The model under review builds one solid part; all positions refer to its coordinate system, in mm. A direction names the side the tool comes from. Coordinates: 2 decimals unless noted, no trailing zeros. Loops run counter-clockwise (first coordinate to the right, second up) from the corner with the lowest first, then second, coordinate; pieces in that order, holes last. Notation, with made-up numbers: M 83,36.25 L 134,36.25 A35 cw 134,74.25 Z; hole C 45.5,62.5 d6. An arc over 180 degrees is marked long. Write item = value, one per line. Start each with the question number.
Q1. We need section B-B on x = 0. Count the separate pieces of the cut face and the enclosed holes in it, and give its area (3 significant figures).
Q2. We need section C-C on y = 26. Give the boundary of the cut face in (x, z), and give its area (3 significant figures).
Q3. Mouldability with a two-part tool opening along X and no side actions: class faces 4 (the face through (-1.11, 16.01, 1.27)), 5 (the face through (-5, 15, 2)), 6 (the face through (0, 0, 1)) as released by +X, released by -X, zero draft, split by the parting line, or undercut.
Q4. For faces 1 (the face through (0, 9, 2.5)), 2 (the face through (5, 15, 2)), 3 (the face through (-0.03, 2.25, 1.27)), list the 3-axis set-ups (+Z, -Z, +X, -X, +Y, -Y) from which the entire face can be reached by the end or side of a thin tool; tool diameter is ignored.
Q5. Wall thickness on probe 1 along Y at (x, z) = (0, 1.85); probe 2 along Y at (x, z) = (0, 0.95); probe 3 along Z at (x, y) = (3, 11): over which ranges is each line inside the solid? List them lowest first.
Q6. Clearance check with flat-ended pins moving along their axes: pin 1 Ø4 at (x, y) = (1.5, 7.5) entering from +Z; pin 2 Ø2 at (x, y) = (-3.5, 21.5) entering from -Z. State where each tip first meets the part, or that it passes through.
Q7. We need section D-D on z = 7.5. Give the boundary of the cut face in (x, y), and give its area (3 significant figures).
Q8. We need section A-A on y = 15. Give the boundary of the cut face in (x, z), and give its area (3 significant figures).
from build123d import *

# Parameters (mm, degrees)
F1_DEPTH      = 5
F1_DEPTH_BACK = 5
F2_R          = 3
F3_R          = 3
F4_R          = 1.5
F5_DEPTH      = 2.5


with BuildPart() as f1:
    # F0 (on Right) → F1 (new body, two sides)
    with BuildSketch(Plane.YZ) as f1_sk:
        Polygon((0, 2.5), (0, 0), (21, 0), (24, 4), (22, 5.5), (19.75, 2.5), align=None)
        Polygon((22, 5.5), (24, 4), (30, 6), (29.209430585, 8.3717082451), (22.4685647168, 6.1247529557), align=None)
    extrude(amount=F1_DEPTH)
    extrude(f1_sk.sketch, amount=-F1_DEPTH_BACK)

    # F2
    f2_edges = [f1.edges().sort_by_distance(p)[0] for p in [
        (0, 21, 0),
        (0, 19.75, 2.5),
    ]]
    fillet(f2_edges, radius=F2_R)

    # F3
    f3_edges = [f1.edges().sort_by_distance(p)[0] for p in [
        (0, 22.468565, 6.124753),
        (0, 24, 4),
    ]]
    fillet(f3_edges, radius=F3_R)

    # F4 (on face) → F5 (cut, through all)
    with BuildSketch(Plane.XY.offset(2.5)):
        with Locations((0, 15)):
            Circle(F4_R)
        with BuildLine():
            ThreePointArc((1.4947825929, 3.875), (1.4986950806, 3.937445581), (1.5, 4))
            ThreePointArc((1.5, 4), (1.4986950806, 4.062554419), (1.4947825929, 4.125))
            ThreePointArc((1.4947825929, 4.125), (1.4882142436, 4.0623344324), (1.4790199458, 4))
            ThreePointArc((1.4790199458, 4), (1.4882142436, 3.9376655676), (1.4947825929, 3.875))
        make_face()
        with BuildLine():
            ThreePointArc((-1.4790199458, 4), (-1.4882142436, 4.0623344324), (-1.4947825929, 4.125))
            ThreePointArc((-1.4947825929, 4.125), (-1.4986950806, 4.062554419), (-1.5, 4))
            ThreePointArc((-1.5, 4), (-1.4986950806, 3.937445581), (-1.4947825929, 3.875))
            ThreePointArc((-1.4947825929, 3.875), (-1.4882142436, 3.9376655676), (-1.4790199458, 4))
        make_face()
        with BuildLine():
            ThreePointArc((-1.4790199458, 4), (0, 2.75), (1.4790199458, 4))
            ThreePointArc((1.4790199458, 4), (0, 5.25), (-1.4790199458, 4))
        make_face()
        with BuildLine():
            ThreePointArc((1.4790199458, 4), (1.4882142436, 4.0623344324), (1.4947825929, 4.125))
            ThreePointArc((1.4947825929, 4.125), (0, 5.5), (-1.4947825929, 4.125))
            ThreePointArc((-1.4947825929, 4.125), (-1.4882142436, 4.0623344324), (-1.4790199458, 4))
            ThreePointArc((-1.4790199458, 4), (0, 5.25), (1.4790199458, 4))
        make_face()
        with BuildLine():
            ThreePointArc((-1.4947825929, 4.125), (0, 5.5), (1.4947825929, 4.125))
            ThreePointArc((1.4947825929, 4.125), (1.4986950806, 4.187445581), (1.5, 4.25))
            ThreePointArc((1.5, 4.25), (0, 5.75), (-1.5, 4.25))
            ThreePointArc((-1.5, 4.25), (-1.4986950806, 4.187445581), (-1.4947825929, 4.125))
        make_face()
        with BuildLine():
            ThreePointArc((-1.4947825929, 3.875), (0, 2.5), (1.4947825929, 3.875))
            ThreePointArc((1.4947825929, 3.875), (1.4882142436, 3.9376655676), (1.4790199458, 4))
            ThreePointArc((1.4790199458, 4), (0, 2.75), (-1.4790199458, 4))
            ThreePointArc((-1.4790199458, 4), (-1.4882142436, 3.9376655676), (-1.4947825929, 3.875))
        make_face()
        with BuildLine():
            ThreePointArc((1.5, 3.75), (1.4986950806, 3.812554419), (1.4947825929, 3.875))
            ThreePointArc((1.4947825929, 3.875), (0, 2.5), (-1.4947825929, 3.875))
            ThreePointArc((-1.4947825929, 3.875), (-1.4986950806, 3.812554419), (-1.5, 3.75))
            ThreePointArc((-1.5, 3.75), (0, 2.25), (1.5, 3.75))
        make_face()
        with BuildLine():
            ThreePointArc((1.4947825929, 4.125), (1.4986950806, 4.062554419), (1.5, 4))
            Line((1.5, 4), (1.5, 4.25))
            ThreePointArc((1.5, 4.25), (1.4986950806, 4.187445581), (1.4947825929, 4.125))
        make_face()
        with BuildLine():
            Line((1.5, 3.75), (1.5, 4))
            ThreePointArc((1.5, 4), (1.4986950806, 3.937445581), (1.4947825929, 3.875))
            ThreePointArc((1.4947825929, 3.875), (1.4986950806, 3.812554419), (1.5, 3.75))
        make_face()
        with BuildLine():
            ThreePointArc((-1.5, 4), (-1.4986950806, 4.062554419), (-1.4947825929, 4.125))
            ThreePointArc((-1.4947825929, 4.125), (-1.4986950806, 4.187445581), (-1.5, 4.25))
            Line((-1.5, 4.25), (-1.5, 4))
        make_face()
        with BuildLine():
            ThreePointArc((-1.5, 3.75), (-1.4986950806, 3.812554419), (-1.4947825929, 3.875))
            ThreePointArc((-1.4947825929, 3.875), (-1.4986950806, 3.937445581), (-1.5, 4))
            Line((-1.5, 4), (-1.5, 3.75))
        make_face()
    extrude(amount=-F5_DEPTH, mode=Mode.SUBTRACT)


solid = f1.part
Returned:
q1.separate_pieces = 3
q1.enclosed_holes = 0
q1.area = 63.4 mm^2
q2.outline = M -5,4.67 L 5,4.67 L 5,7.3 L -5,7.3 Z
q2.area = 26.4 mm^2
q3.face_4 = undercut
q3.face_5 = released by -X
q3.face_6 = zero draft
q4.face_1 = +Z, +X, -X, -Y
q4.face_2 = +Z, -Z, +X, +Y, -Y
q4.face_3 = +Z, -Z
q5.probe_1 = 0 to 2.25, 5.75 to 13.5, 16.5 to 22.39
q5.probe_2 = 0 to 2.25, 5.75 to 13.5, 16.5 to 21.69
q5.probe_3 = 0 to 2.5
q6.pin_1 = 2.5
q6.pin_2 = 0.17
q7.outline = M -5,26.59 L 5,26.59 L 5,29.5 L -5,29.5 Z
q7.area = 29.1 mm^2
q8.outline = M -5,0 L -1.5,0 L -1.5,2.5 L -5,2.5 Z; M 1.5,0 L 5,0 L 5,2.5 L 1.5,2.5 Z
q8.area = 17.5 mm^2
